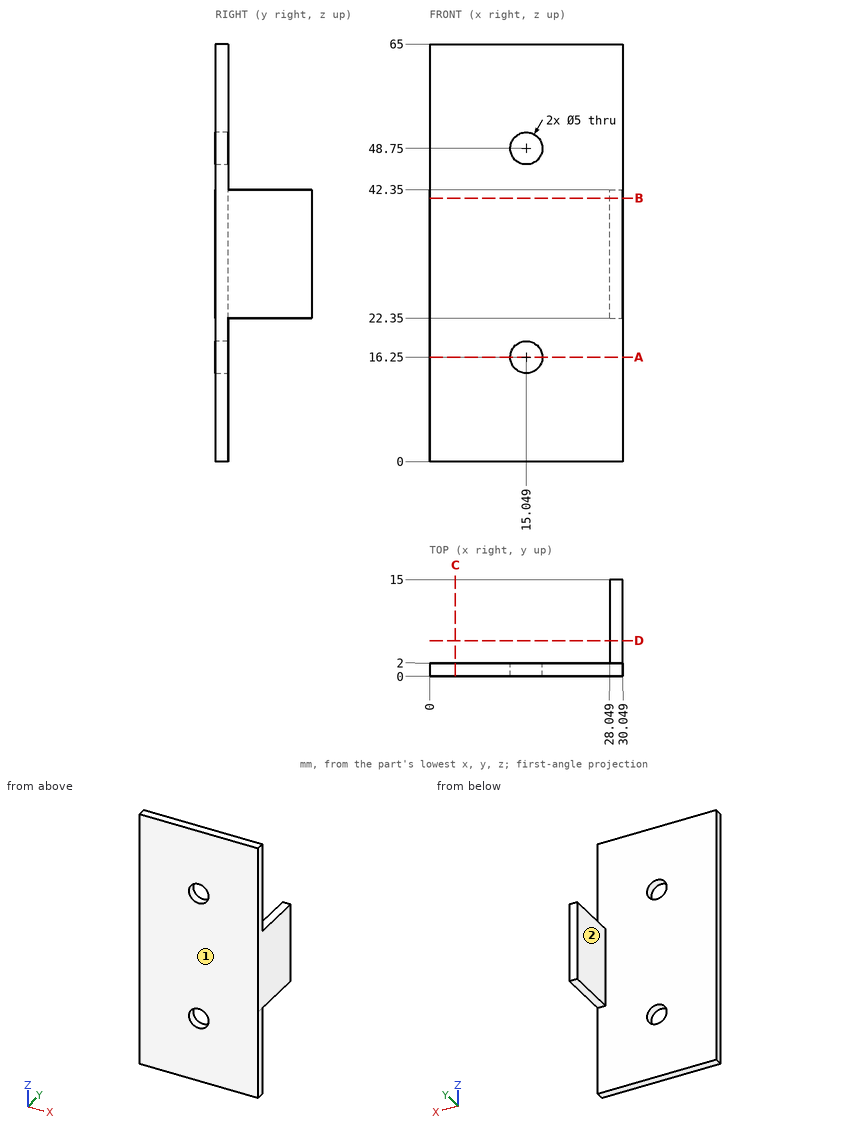
Answer from the drawing. Dimensions are ordinates in mm from the lowest x, y and z of the part. A direction names the side the tool comes from. Give positions to 0.01 mm unless a question says otherwise; leave off trailing zeros. Loops run counter-clockwise (first coordinate to the right, second up) from the corner with the lowest first, then second, coordinate; pieces in that order, holes last. Notation, with made-up numbers: (16, 61) - (73, 61) arc R10 cw to (73, 79) - close; hole circle Ø7 at (-15.5, 89.25). An arc over 180 degrees is marked (long way). Write each question's results on one line, items separated by ' | '.
1. Find section D-D, the plane y = 5.5. Write down the section's boundary in (x, z).
Resolved:
outline: (28.05, 22.35) - (30.05, 22.35) - (30.05, 42.35) - (28.05, 42.35) - close
2. Consider probe 1 along X at (y, z) = (0.4, 16.25); probe 2 along Z at (x, y) = (16, 1); probe 3 along Y at (x, z) = (3, 8.5). Determine where each line is inside the solid, lowest interval first. Write a range as from..to.
Resolved:
probe 1: x = 0..12.55, 17.55..30.05 | probe 2: z = 0..13.94, 18.56..46.44, 51.06..65 | probe 3: y = 0..2
3. Which of the six approach directions +Z, -Z, +X, -X, +Y, -Y give full straight-line access (tool end or side, diameter ignored) to the marked faces 1 and 2?
Resolved:
face 1: +Z, -Z, +X, -X, -Y | face 2: +Z, -Z, -X, +Y
4. Flat-ended cylindrical pins translate along their axes: P1, Ø1, axis at y = 6.5, z = 43.5, coming from the -X side; P2, Ø1, axis at x = 29, y = 7.5, coming from the -Z side; P3, Ø1.6, axis at x = 29, y = 11, coming from the +Z side; P4, Ø10, axis at x = 13, z = 53, coming from the +Y side. Find the tip coordinate at first contact, or state that the pin passes through.
Resolved:
P1: passes through | P2: stops at z = 22.35 | P3: stops at z = 42.35 | P4: stops at y = 2
5. Find section A-A, the plane z = 16.25. Write down the section's boundary in (x, y).
Resolved:
outline: (0, 0) - (12.55, 0) - (12.55, 2) - (0, 2) - close; (17.55, 0) - (30.05, 0) - (30.05, 2) - (17.55, 2) - close
6. Find section B-B, the plane z = 41. Write down the section's boundary in (x, y).
Resolved:
outline: (0, 0) - (30.05, 0) - (30.05, 15) - (28.05, 15) - (28.05, 2) - (0, 2) - close
7. Find section C-C, the plane x = 4. Write down the section's boundary in (y, z), then the cut area to 3 significant figures.
Resolved:
outline: (0, 0) - (2, 0) - (2, 65) - (0, 65) - close | area: 130 mm^2
